Here's how the part is built. I have some questions about the finished solid (model axes, mm). Face numbers are marked on the shaded views. A direction names the side the tool comes from. Give positions to 0.01 mm unless a question says otherwise; leave off trailing zeros. Write each loop counter-clockwise with the first axis right and the second up, starting at its lowest first coordinate (ties: lowest second). Pieces come first, ordered by that corner, then holes. Notation, with made-up numbers: (69, 82.5) - (93, 82.5) arc R23 cw to (93, 121.5) - close; hole circle Ø6 at (9, -5). An arc over 180 degrees is marked (long way). Use a Markdown table: item, result.
```python
from build123d import *

# Parameters (mm, degrees)
BOX764_W           = 148
BOX764_H           = 74
BOX764_DEPTH       = 55
CYLINDER1805_R     = 74
CYLINDER1805_DEPTH = 60
CYLINDER1810_R     = 2.5
CYLINDER1810_DEPTH = 40
CYLINDER1806_R     = 2.5
CYLINDER1806_DEPTH = 40
CYLINDER1885_R     = 2.5
CYLINDER1885_DEPTH = 40
CYLINDER1809_R     = 2.5
CYLINDER1809_DEPTH = 40
BOX769_W           = 10
BOX769_H           = 56
BOX769_DEPTH       = 49
CHAMFER065_SIZE    = 3


with BuildPart() as krychle764:
    # Box764 → Box764 (new body)
    with BuildSketch(Plane(origin=(-74, 0, 29), x_dir=(1, 0, 0), z_dir=(0, 0, 1))):
        with Locations((74, 37)):
            Rectangle(BOX764_W, BOX764_H)
    extrude(amount=BOX764_DEPTH)


with BuildPart() as obj1:
    # Cylinder1805 → Cylinder1805 (new body)
    with BuildSketch(Plane.XY.offset(26)):
        Circle(CYLINDER1805_R)
    extrude(amount=CYLINDER1805_DEPTH)


with BuildPart() as obj2:
    # Cylinder1810 → Cylinder1810 (new body)
    with BuildSketch(Plane(origin=(-86, 20, 39), x_dir=(0, 0, -1), z_dir=(1, 0, 0))):
        Circle(CYLINDER1810_R)
    extrude(amount=CYLINDER1810_DEPTH)


with BuildPart() as obj3:
    # Cylinder1806 → Cylinder1806 (new body)
    with BuildSketch(Plane(origin=(-86, -10, 69), x_dir=(0, 0, -1), z_dir=(1, 0, 0))):
        Circle(CYLINDER1806_R)
    extrude(amount=CYLINDER1806_DEPTH)


with BuildPart() as obj4:
    # Cylinder1885 → Cylinder1885 (new body)
    with BuildSketch(Plane(origin=(-86, 16, 68), x_dir=(0, 0, -1), z_dir=(1, 0, 0))):
        Circle(CYLINDER1885_R)
    extrude(amount=CYLINDER1885_DEPTH)


with BuildPart() as compound919:
    # Cylinder1809 → Cylinder1809 (new body)
    with BuildSketch(Plane(origin=(-86, -10, 39), x_dir=(0, 0, -1), z_dir=(1, 0, 0))):
        Circle(CYLINDER1809_R)
    extrude(amount=CYLINDER1809_DEPTH)

    # Compound919: union obj2, obj3, obj4
    add(obj2.part)
    add(obj3.part)
    add(obj4.part)


with BuildPart() as cut568:
    # Box769 → Box769 (new body)
    with BuildSketch(Plane(origin=(-79, -24, 29), x_dir=(1, 0, 0), z_dir=(0, 0, 1))):
        with Locations((5, 28)):
            Rectangle(BOX769_W, BOX769_H)
    extrude(amount=BOX769_DEPTH)

    # Chamfer065
    chamfer065_edges = [cut568.edges().sort_by_distance(p)[0] for p in [
        (-79, 32, 53.5),
    ]]
    chamfer(chamfer065_edges, length=CHAMFER065_SIZE)

    # Cut556: cut Compound919
    add(compound919.part, mode=Mode.SUBTRACT)

    # Cut557: cut obj1
    add(obj1.part, mode=Mode.SUBTRACT)

    # Cut568: cut Krychle764
    add(krychle764.part, mode=Mode.SUBTRACT)


solid = cut568.part
```
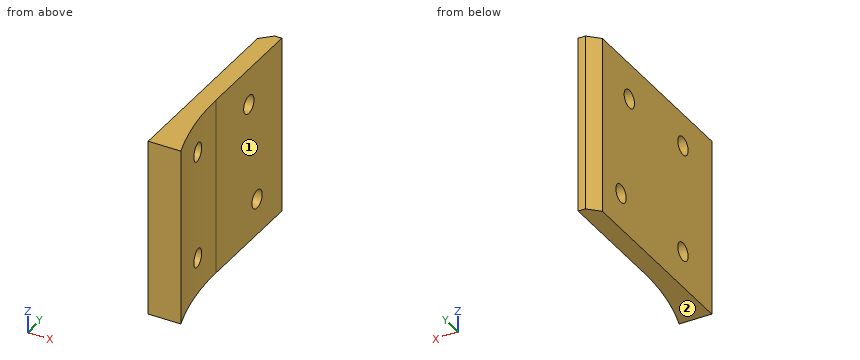
Item 1: Will this pin go through, and if not, where does the flat tip stop? pin 1 Ø2 at (y, z) = (11, 52.5) entering from +X.
Values:
| item | result |
|---|---|
| pin 1 | stops at x = -74 |
Item 2: I need wall thicknesses on line 1 along Y through (x, z) = (-76, 39); line 2 along Z through (x, y) = (-77, -10); line 3 along Y through (x, z) = (-76.95, 68). Which ranges of each line are inside material? Lowest first, please. Write a range as [from, to].
Values:
| item | result |
|---|---|
| line 1 | y = [-24, -12.5], [-7.5, 17.5], [22.5, 32] |
| line 2 | z = [29, 36.5], [41.5, 66.5], [71.5, 78] |
| line 3 | y = [-24, -12.29], [-7.71, 13.5], [18.5, 31.05] |
Item 3: If we section it at C-C, the plane y = -10: Write out the boundary of the cut face in (x, z), plus the area to 3 significant figures.
Values:
| item | result |
|---|---|
| outline | (-79, 29) - (-73.32, 29) - (-73.32, 36.5) - (-79, 36.5) - close; (-79, 41.5) - (-73.32, 41.5) - (-73.32, 66.5) - (-79, 66.5) - close; (-79, 71.5) - (-73.32, 71.5) - (-73.32, 78) - (-79, 78) - close |
| area | 221 mm2 |
Item 4: If we section it at B-B, the plane z = 68: Write out the boundary of the cut face in (x, y), plus the area to 3 significant figures.
Values:
| item | result |
|---|---|
| outline | (-79, -24) - (-70, -24) arc R74 cw to (-72.97, -12.29) - (-79, -12.29) - close; (-79, -7.71) - (-73.6, -7.71) arc R74 cw to (-74, 0) - (-74, 13.5) - (-79, 13.5) - close; (-79, 18.5) - (-74, 18.5) - (-74, 32) - (-76, 32) - (-79, 29) - close |
| area | 256 mm2 |
Item 5: For the marked faces 1 and 2, which set-ups out of +Z, -Z, +X, -X, +Y, -Y let a thin tool reach every point of the face, with its end or its side?
Values:
| item | result |
|---|---|
| face 1 | +Z, -Z, +X, +Y |
| face 2 | -Z, +X, -X, +Y, -Y |
Item 6: If we section it at A-A, the plane y = 16: Write out the boundary of the cut face in (x, z), plus the area to 3 significant figures.
Values:
| item | result |
|---|---|
| outline | (-79, 29) - (-74, 29) - (-74, 65.5) - (-79, 65.5) - close; (-79, 70.5) - (-74, 70.5) - (-74, 78) - (-79, 78) - close |
| area | 220 mm2 |
Item 7: If we section it at D-D, the plane z = 45.5: Write out the boundary of the cut face in (x, y).
Values:
| item | result |
|---|---|
| outline | (-79, -24) - (-70, -24) arc R74 cw to (-74, 0) - (-74, 32) - (-76, 32) - (-79, 29) - close |
